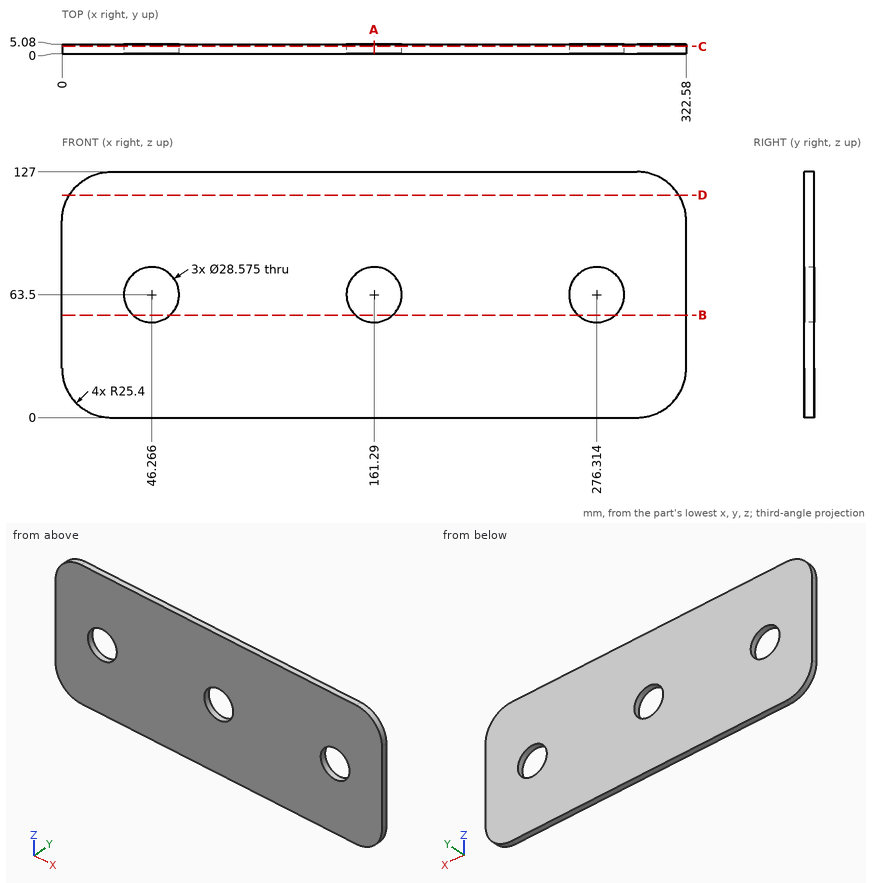
Geometry check sheet. Reference: drawing and pictorial views, mm from the part's lowest x, y, z. Round coordinates to 2 decimals unless told otherwise and drop trailing zeros. Order: outer loops, then holes, each group sorted by start corner. A loop starts at its lowest first (then second) coordinate and runs counter-clockwise, first axis right, second up.
Q1. Cross-section at B-B, the plane z = 53. Enter the section's corners in (x, y), plus the area to 3 significant figures.
Filled sheet:
outline: (0, 0) - (36.58, 0) - (36.58, 5.08) - (0, 5.08) - close; (55.96, 0) - (151.6, 0) - (151.6, 5.08) - (55.96, 5.08) - close; (170.98, 0) - (266.62, 0) - (266.62, 5.08) - (170.98, 5.08) - close; (286, 0) - (322.58, 0) - (322.58, 5.08) - (286, 5.08) - close
area: 1,340 mm2
Q2. Cross-section at C-C, the plane y = 3.9. Enter the section's corners in (x, z) (1 decimal).
Filled sheet:
outline: (0, 25.4) arc R25.4 ccw to (25.4, 0) - (297.2, 0) arc R25.4 ccw to (322.6, 25.4) - (322.6, 101.6) arc R25.4 ccw to (297.2, 127) - (25.4, 127) arc R25.4 ccw to (0, 101.6) - close; hole circle Ø28.6 at (46.3, 63.5); hole circle Ø28.6 at (161.3, 63.5); hole circle Ø28.6 at (276.3, 63.5)
Q3. Cross-section at A-A, the plane x = 161.29. Enter the section's corners in (y, z).
Filled sheet:
outline: (0, 0) - (5.08, 0) - (5.08, 49.21) - (0, 49.21) - close; (0, 77.79) - (5.08, 77.79) - (5.08, 127) - (0, 127) - close
Q4. Scan lines: L1, parallel to Z at x = 161.29, y = 3.95; L2, parallel to Z at x = 173.5, y = 4.05; L3, parallel to X at y = 3.3, z = 116. Record each from-to range of solid material in increasing order.
Filled sheet:
L1: z = 0 to 49.21, 77.79 to 127
L2: z = 0 to 56.08, 70.92 to 127
L3: x = 4.48 to 318.1
Q5. Cross-section at D-D, the plane z = 115. Enter the section's corners in (x, y), plus the area to 3 significant figures.
Filled sheet:
outline: (3.82, 0) - (318.76, 0) - (318.76, 5.08) - (3.82, 5.08) - close
area: 1,600 mm2
